Autodesk Inventor part; units mm, degrees
ref_plane "YZ Plane" through (0, 0, 0) normal (1, 0, 0) x (0, 1, 0)
ref_plane "XZ Plane" through (0, 0, 0) normal (0, 1, 0) x (-1, 0, 0)
ref_plane "XY Plane" through (0, 0, 0) normal (0, 0, 1) x (1, 0, 0)
sketch "Sketch1" plane through (0, 0, 0) normal (1, 0, 0) x (0, 1, 0)
  line L0 (0, 0) -> (0, -125)
  arc A0 (0, -125) -> (3.9145, -123.4868) centre (-11.1642, -90.2991) ccw
  arc A1 (12.4221, -111.3025) -> (14.7058, -62.5) centre (-60.3675, -83.4416) ccw
  line L1 (0, 0) -> (16.1672, -68.711)
  arc A2 (3.9145, -123.4868) -> (12.4221, -111.3025) centre (-26.7088, -93.042) ccw
  dimension "d0" = 125
extrude "Extrusion1" add sketch "Sketch1" along normal blind 600 contours L1 A1 A2 A0 L0
sketch "Sketch2" plane through (0, 0, 0) normal (-1, 0, 0) x (0, 0, 1)
  line L0 (0, 0) -> (-125, 0)
  line L1 (-89.759, 17.1606) -> (-81.759, 17.1606)
  line L2 (-81.759, 17.1606) -> (-81.759, 9.1606)
  line L3 (-81.759, 9.1606) -> (-89.759, 9.1606)
  line L4 (-89.759, 9.1606) -> (-89.759, 17.1606)
  line L5 (-89.759, 17.1606) -> (-81.759, 9.1606) construction
  line L6 (-81.759, 17.1606) -> (-89.759, 9.1606) construction
  dimension "d3" = 8
  dimension "d4" = 8
extrude "Extrusion2" add sketch "Sketch2" along normal blind 48
sketch "Sketch3" plane through (0, 9.1606, -89.759) normal (0, -1, 0) x (1, 0, 0)
  point P0 (0, 89.759)
sketch "Sketch4" plane through (0, 0, 0) normal (0, 0.9734, 0.229) x (1, 0, 0)
  point P0 (0, 0)
sketch "Sketch5" plane through (0, 9.1606, -89.759) normal (0, -1, 0) x (1, 0, 0)
  line L0 (0, 0) -> (-48, 0)
  line L1 (0, 0) -> (-39, 0)
  line L2 (-39, 0) -> (-39, 4)
  line L3 (-39, 4) -> (0, 4)
  line L4 (0, 4) -> (0, 0)
  circle A0 centre (-39, 4) radius 24
  circle A1 centre (-39, 4) radius 5
  point P0 (0, 89.759)
  dimension "d7" = 39
  dimension "d8" = 4
  dimension "d9" = 48
  dimension "d12" = 10
extrude "Extrusion3" add sketch "Sketch5" against normal blind 8 contours A0 L3 A1 L0 | L0 A1 L3 A0 | A1 L0 | L0 L2 L3 A1 | L0 A1 L3 L2
sketch "Sketch6" plane through (0, 17.1606, -81.759) normal (0, 1, 0) x (1, 0, 0)
  point P0 (0, -81.759)
sketch "Sketch7" plane through (0, 9.1606, -89.759) normal (0, -1, 0) x (1, 0, 0)
  point P0 (0, 89.759)
sketch "Sketch8" plane through (0, 9.1606, -89.759) normal (0, -1, 0) x (1, 0, 0)
  line L0 (0, 8) -> (0, 0)
  line L1 (0, 0) -> (-39, 0)
  line L2 (-39, 0) -> (-39, 4)
  line L3 (-39, 4) -> (0, 4)
  line L4 (0, 4) -> (0, 0)
  circle A0 centre (-39, 4) radius 5
  point P0 (0, 89.759)
  dimension "d13" = 39
  dimension "d14" = 4
  dimension "d15" = 10
extrude "Extrusion4" cut sketch "Sketch8" against normal blind 8 contours A0 L1 L2 L3 | L3 L2 L1 A0
properties part number "R wing"
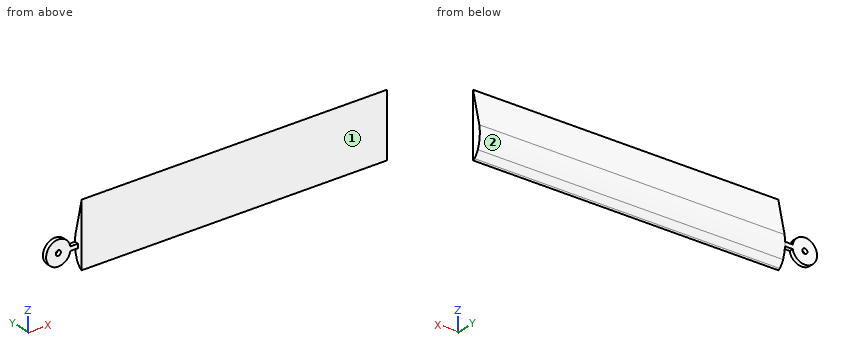
Geometry check sheet. Reference: the model listing, model coordinates, mm. Face numbers are marked on the shaded views. A direction names the side the tool comes from. Coordinates: 2 decimals unless noted, no trailing zeros. Order: outer loops, then holes, each group sorted by start corner. A loop starts at its lowest first (then second) coordinate and runs counter-clockwise, first axis right, second up.
Q1. Sectioned sample at B-B on z = -47. Record the cut outline in (x, y), and give its area (3 significant figures).
Reply:
outline: (0, 0) - (600, 0) - (600, 11.06) - (0, 11.06) - close
area: 6,640 mm2
Q2. Sectioned sample at A-A on x = 437. Record the cut outline in (y, z).
Reply:
outline: (0, -125) arc R36.45 ccw to (3.91, -123.49) arc R43.18 ccw to (12.42, -111.3) arc R77.94 ccw to (16.17, -68.71) - (0, 0) - close
Q3. Tool access check on the marked faces 1 and 2. Record the directions out of +Z, -Z, +X, -X, +Y, -Y that give a thin tool (end or side, any length) a straight path to the whole face; none if there is none.
Reply:
face 1: +Z, -Z, +X, -X, -Y
face 2: +X, +Y
Q4. Thickness scan on probe 1 along Z at (x, y) = (-39, 13.75); probe 2 along X at (y, z) = (7.75, -64); probe 3 along X at (y, z) = (16.5, -88.5). Record the ranges inside material, lowest first.
Reply:
probe 1: z = -109.76 to -90.76, -80.76 to -61.76
probe 2: x = 0 to 600
probe 3: x = -62.84 to -43.18, -34.82 to 600
Q5. Depth check by flat-ended pin: pin 1 Ø3 at (x, y) = (514, 3) entering from -Z; pin 2 Ø8 at (x, y) = (285, 9.5) entering from -Z; pin 3 Ø10 at (x, y) = (414, 4.5) entering from -Z; pin 4 Ø3 at (x, z) = (130.5, -54.5) entering from +Y. Enter the tip coordinate at first touch or a pass-through.
Reply:
pin 1: stops at z = -124.48
pin 2: stops at z = -121.8
pin 3: stops at z = -125
pin 4: stops at y = 13.18
